Autodesk Inventor part; units mm, degrees
ref_plane "YZ Plane" through (0, 0, 0) normal (1, 0, 0) x (0, 1, 0)
ref_plane "XZ Plane" through (0, 0, 0) normal (0, 1, 0) x (-1, 0, 0)
ref_plane "XY Plane" through (0, 0, 0) normal (0, 0, 1) x (1, 0, 0)
sketch "スケッチ1" plane through (0, 0, 0) normal (0, 0, 1) x (1, 0, 0)
  line L0 (7.5, 15) -> (-7.5, 15)
  line L1 (-7.5, 15) -> (-7.5, -15)
  line L2 (-7.5, -15) -> (7.5, -15)
  line L3 (7.5, -15) -> (7.5, 15)
  line L4 (7.5, 15) -> (-7.5, -15) construction
  line L5 (-7.5, 15) -> (7.5, -15) construction
  line L6 (-5.5, 13) -> (5.5, 13)
  line L7 (5.5, 13) -> (5.5, -13)
  line L8 (5.5, -13) -> (-5.5, -13)
  line L9 (-5.5, -13) -> (-5.5, 13)
  point P0 (0, 0)
  dimension "d0" = 15
  dimension "d1" = 30
  dimension "d2" = 2
extrude "押し出し1" add sketch "スケッチ1" along normal blind 490
sketch "スケッチ2" plane through (-7.5, 15, 0) normal (0, 1, 0) x (1, 0, 0)
  circle A0 centre (7.5, -10) radius 1.6
  circle A1 centre (7.5, -25) radius 1.6
  circle A2 centre (7.5, -480) radius 1.6
  circle A3 centre (7.5, -465) radius 1.6
  line L0 (15, 0) -> (0, 0)
  line L1 (15, -490) -> (0, -490)
  circle A4 centre (7.5, -195) radius 1.6
  circle A5 centre (7.5, -210) radius 1.6
  point P0 (7.5, 0)
  point P1 (7.5, 0)
  dimension "d5" = 3.2
  dimension "d6" = 3.2
  dimension "d7" = 3.2
  dimension "d8" = 3.2
  dimension "d9" = 10
  dimension "d10" = 15
  dimension "d11" = 10
  dimension "d12" = 15
  dimension "d15" = 3.2
  dimension "d16" = 3.2
  dimension "d17" = 15
  dimension "d18" = 170
extrude "押し出し2" cut sketch "スケッチ2" against normal through all
sketch "スケッチ3" plane through (7.5, -15, 0) normal (1, 0, 0) x (0, 0, -1)
  circle A0 centre (-50, 22.5) radius 1.6
  circle A1 centre (-60, 22.5) radius 1.6
  circle A2 centre (-70, 22.5) radius 1.6
  line L0 (0, 30) -> (-490, 30)
  circle A3 centre (-350, 22.5) radius 1.6
  circle A4 centre (-360, 22.5) radius 1.6
  circle A5 centre (-370, 22.5) radius 1.6
  point P0 (0, 15)
  dimension "d19" = 3.2
  dimension "d20" = 3.2
  dimension "d21" = 3.2
  dimension "d22" = 7.5
  dimension "d23" = 50
  dimension "d24" = 10
  dimension "d25" = 10
  dimension "d26" = 3.2
  dimension "d27" = 3.2
  dimension "d28" = 3.2
  dimension "d29" = 10
  dimension "d30" = 10
  dimension "d31" = 300
extrude "押し出し3" cut sketch "スケッチ3" against normal through all
properties part number "オムニ_角柱3" material "アルミニウム 6061"
The listing builds one solid part. Answer for the finished solid, in the listing's coordinates (mm). A direction names the side the tool comes from. Give positions to 0.01 mm unless a question says otherwise; leave off trailing zeros. Order: outer loops, then holes, each group sorted by start corner. A loop starts at its lowest first (then second) coordinate and runs counter-clockwise, first axis right, second up.
Item 1: The part is cut by section B-B, the plane z = 217.5. Give the vertices of the cut face in (x, y).
From the geometry:
outline: (-7.5, -15) - (7.5, -15) - (7.5, 15) - (-7.5, 15) - close; hole (-5.5, -13) - (5.5, -13) - (5.5, 13) - (-5.5, 13) - close
Item 2: Which of the six approach directions +Z, -Z, +X, -X, +Y, -Y give full straight-line access (tool end or side, diameter ignored) to faces 1 (the face through (0, -13, 242)), 2 (the face through (-7, 0, 490))?
From the geometry:
face 1: +Z, -Z
face 2: +Z, +X, -X, +Y, -Y
Item 3: For a pull along X with two mould halves and no side action, classify faces 3 (the face through (7.5, 0, 242)), 4 (the face through (0, 15, 242)), 5 (the face through (0, 13, 242)) as pulls with the +X half, pulls with the -X half, needs draft (parallel to the pull), parting line crosses it, or undercut.
From the geometry:
face 3: pulls with the +X half
face 4: needs draft
face 5: undercut
Item 4: Find the intervals of material crossed by probe 1 along X at (y, z) = (-5.25, 333); probe 2 along Y at (x, z) = (-2.75, 68.5); probe 3 along Y at (x, z) = (-6.2, 60), in increasing order.
From the geometry:
probe 1: x = -7.5 to -5.5, 5.5 to 7.5
probe 2: y = -15 to -13, 13 to 15
probe 3: y = -15 to 5.9, 9.1 to 15
Item 5: Given pin 1 Ø1.9 at (y, z) = (7.5, 350) entering from -X; pin 2 Ø4 at (x, z) = (0, 210) entering from -Y, each flat-ended and moving along its own axis, determine where each tip first touches the part or whether it passes through.
From the geometry:
pin 1: passes through
pin 2: stops at y = -15
Item 6: The part is cut by section A-A, the plane y = -7.25. Give the vertices of the cut face in (x, z).
From the geometry:
outline: (-7.5, 0) - (-5.5, 0) - (-5.5, 490) - (-7.5, 490) - close; (5.5, 0) - (7.5, 0) - (7.5, 490) - (5.5, 490) - close
